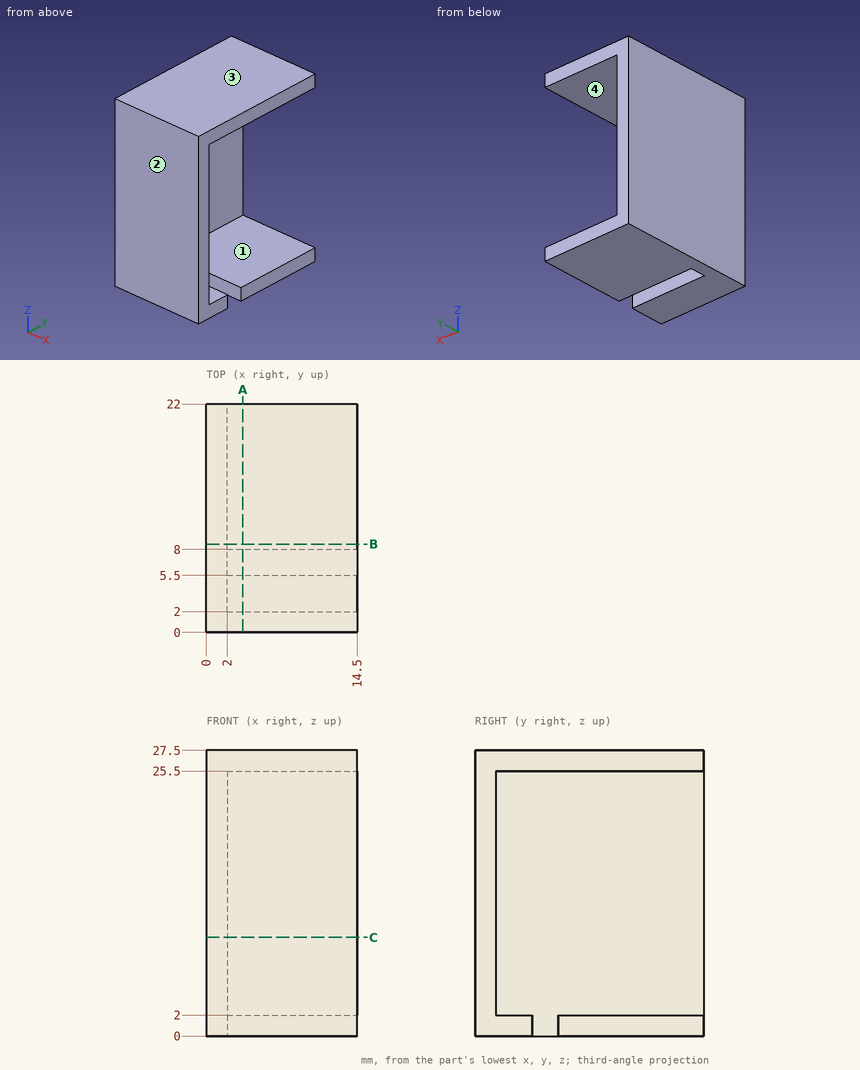
For this review, use the dimensioned drawing (mm, ordinates from the lowest corner) and the shaded views. Coordinates: 2 decimals unless noted, no trailing zeros. Loops run counter-clockwise (first coordinate to the right, second up) from the corner with the lowest first, then second, coordinate; pieces in that order, holes last. Notation, with made-up numbers: (-5.5, -13) -> (-1.5, -13) arc R27 cw to (-1.5, 6) -> close; hole circle Ø5 at (15, 69). An arc over 180 degrees is marked (long way). Return JSON: item names as keys, results as strings. Group by question number.
(1) Consider section C-C, the plane z = 9.5. Give the boundary of the cut face in (x, y).
(2) Mouldability with a two-part tool opening along Z and no side actions: class the marked faces 1, 2, 3 and 4 as pulls with the +Z half, pulls with the -Z half, needs draft (parallel to the pull), parting line crosses it, or undercut.
(3) Consider section A-A, the plane x = 3.5. Give the boundary of the cut face in (y, z).
(4) For pin 1 Ø6 at (y, z) = (12.5, 19) entering from +X; pin 2 Ø3 at (x, z) = (12.5, 13.5) entering from +Y, all flat-tipped, find the tip position at first contact; note any pin that passes through.
(5) To check wall thickness, follow L1, parallel to Z at x = 6.5, y = 15; L2, parallel to X at y = 3.75, z = 18.25; L3, parallel to Y at x = 6.75, z = 1.5. State the ranges of each line that lie inside material, in increasing order.
(6) Consider section B-B, the plane y = 8.5. Give the boundary of the cut face in (x, z), plus the area to 3 significant figures.
Results below:
{
 "1": {"outline": "(0, 0) -> (14.5, 0) -> (14.5, 2) -> (2, 2) -> (2, 22) -> (0, 22) -> close"},
 "2": {"face 1": "undercut", "face 2": "needs draft", "face 3": "pulls with the +Z half", "face 4": "undercut"},
 "3": {"outline": "(0, 0) -> (5.5, 0) -> (5.5, 2) -> (2, 2) -> (2, 25.5) -> (22, 25.5) -> (22, 27.5) -> (0, 27.5) -> close; (8, 0) -> (22, 0) -> (22, 2) -> (8, 2) -> close"},
 "4": {"pin 1": "stops at x = 2", "pin 2": "stops at y = 2"},
 "5": {"L1": "z = 0 to 2, 25.5 to 27.5", "L2": "x = 0 to 2", "L3": "y = 0 to 5.5, 8 to 22"},
 "6": {"outline": "(0, 0) -> (14.5, 0) -> (14.5, 2) -> (2, 2) -> (2, 25.5) -> (14.5, 25.5) -> (14.5, 27.5) -> (0, 27.5) -> close", "area": "105 mm2"}
}
